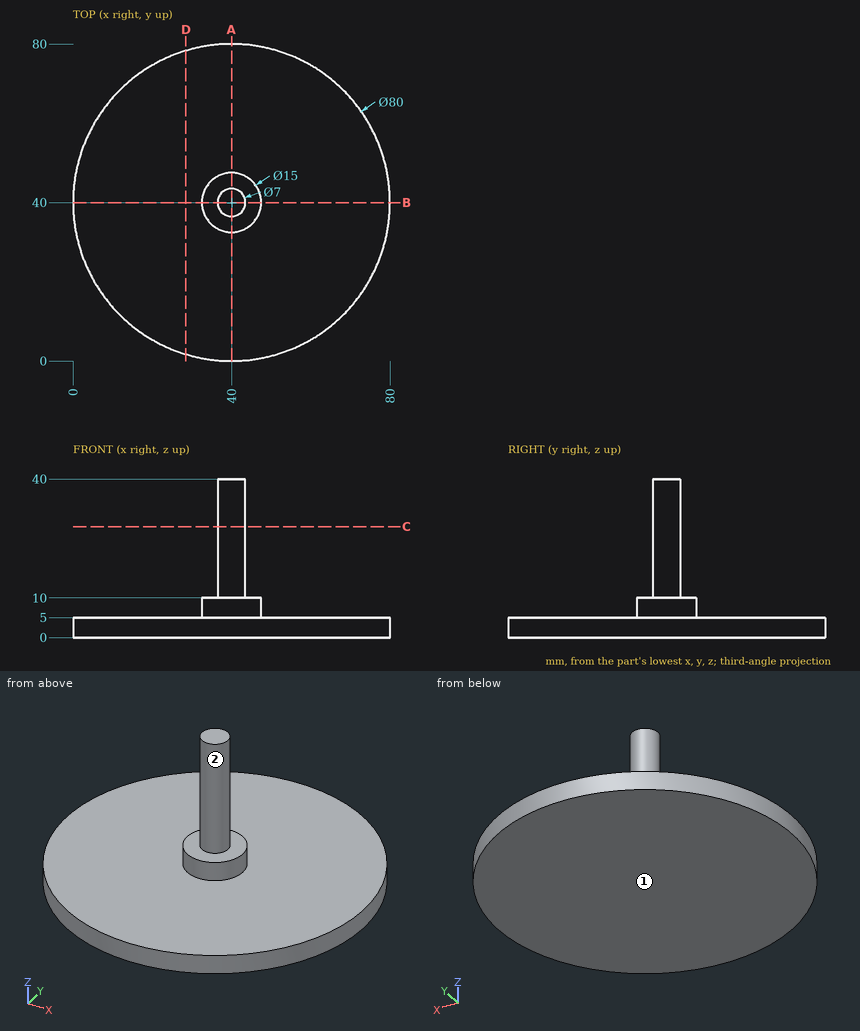
Could you check a few things on this drawing? It's one solid part, dimensions in mm from its lowest x, y, z. A direction names the side the tool comes from. Give positions to 0.01 mm unless a question says otherwise; leave off trailing zeros. Order: outer loops, then holes, each group sorted by start corner. A loop starts at its lowest first (then second) coordinate and runs counter-clockwise, first axis right, second up. Notation, with made-up numbers: (-9, 23) - (26, 23) arc R22 cw to (26, 51) - close; hole circle Ø3 at (30, -24.5). An arc over 180 degrees is marked (long way). Return JSON: item names as keys, results as strings. Group by question number.
Q1. Which directions (+Z, -Z, +X, -X, +Y, -Y) give clear straight access to the entire face, cutting with the end or side of a thin tool? Please do the marked faces 1 and 2.
Q2. Suppose I cut it at A-A, the plane x = 40. Please give me the cut outline in (y, z).
Q3. Please list where these lines run through material, in increasing order: line 1 along Z through (x, y) = (31.5, 14); line 2 along X through (y, z) = (62, 2); line 3 along Y through (x, z) = (42.5, 12). Write a range as [from, to].
Q4. Will these pins go through, and if not, where does the flat tip stop? pin 1 Ø2 at (x, y) = (60, 44.5) entering from +Z; pin 2 Ø3 at (x, z) = (46.5, 31) entering from -Y; pin 3 Ø6 at (x, y) = (56, 56) entering from -Z.
Q5. Suppose I cut it at D-D, the plane x = 28.5. Please give me the cut outline in (y, z).
Q6. Suppose I cut it at C-C, the plane z = 28. Please give me the cut outline in (x, y).
Resolved:
{
 "1": {"face 1": "-Z, +X, -X, +Y, -Y", "face 2": "+Z"},
 "2": {"outline": "(0, 0) - (80, 0) - (80, 5) - (47.5, 5) - (47.5, 10) - (43.5, 10) - (43.5, 40) - (36.5, 40) - (36.5, 10) - (32.5, 10) - (32.5, 5) - (0, 5) - close"},
 "3": {"line 1": "z = [0, 5]", "line 2": "x = [6.59, 73.41]", "line 3": "y = [37.55, 42.45]"},
 "4": {"pin 1": "stops at z = 5", "pin 2": "passes through", "pin 3": "stops at z = 0"},
 "5": {"outline": "(1.69, 0) - (78.31, 0) - (78.31, 5) - (1.69, 5) - close"},
 "6": {"outline": "circle Ø7 at (40, 40)"}
}
